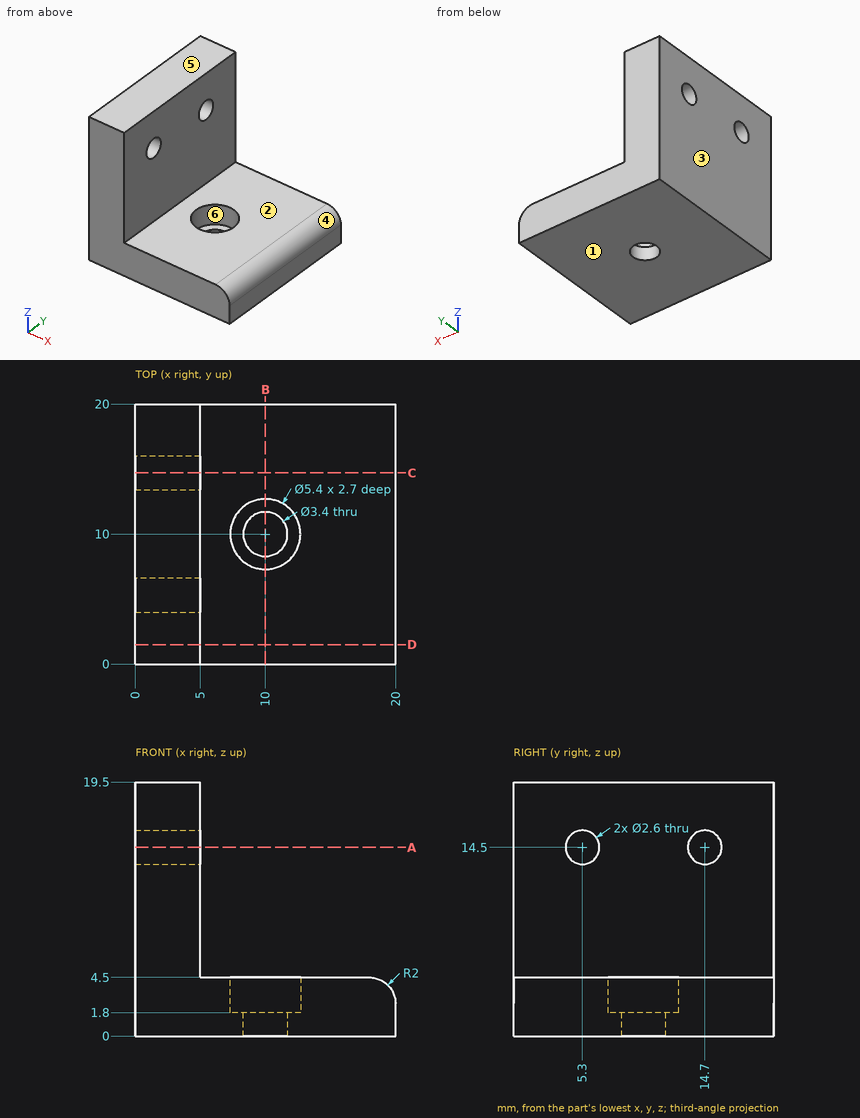
Answer from the drawing. Dimensions are ordinates in mm from the lowest x, y and z of the part. A direction names the side the tool comes from. Round coordinates to 2 decimals unless told otherwise and drop trailing zeros. Write each loop counter-clockwise with the first axis right and the second up, starting at its lowest first coordinate (ties: lowest second). Pieces come first, ordered by that corner, then holes. Notation, with made-up numbers: (-21, 67) - (0, 67) arc R29 cw to (0, 98) - close; hole circle Ø3 at (7, 48.25). An arc over 180 degrees is marked (long way). Use a Markdown table: item, result.
(1) Which of the six approach directions +Z, -Z, +X, -X, +Y, -Y give full straight-line access (tool end or side, diameter ignored) to the marked faces 1 and 2?
Reported:
| item | result |
|---|---|
| face 1 | -Z, +X, -X, +Y, -Y |
| face 2 | +Z, +X, +Y, -Y |
(2) The mould has two halves that part along X. Classify the marked faces 3, 4, 5 and 6: released by +X, released by -X, zero draft, split by the parting line, or undercut.
Reported:
| item | result |
|---|---|
| face 3 | released by -X |
| face 4 | released by +X |
| face 5 | zero draft |
| face 6 | undercut |
(3) The part is cut by section A-A (z = 14.5). Write down the section's boundary in (x, y).
Reported:
| item | result |
|---|---|
| outline | (0, 0) - (5, 0) - (5, 4) - (0, 4) - close; (0, 6.6) - (5, 6.6) - (5, 13.4) - (0, 13.4) - close; (0, 16) - (5, 16) - (5, 20) - (0, 20) - close |
(4) The part is cut by section D-D (y = 1.5). Write down the section's boundary in (x, z), then the cut area to 3 significant figures.
Reported:
| item | result |
|---|---|
| outline | (0, 0) - (20, 0) - (20, 2.5) arc R2 ccw to (18, 4.5) - (5, 4.5) - (5, 19.5) - (0, 19.5) - close |
| area | 164 mm2 |
(5) The part is cut by section B-B (x = 10). Write down the section's boundary in (y, z).
Reported:
| item | result |
|---|---|
| outline | (0, 0) - (8.3, 0) - (8.3, 1.8) - (7.3, 1.8) - (7.3, 4.5) - (0, 4.5) - close; (11.7, 0) - (20, 0) - (20, 4.5) - (12.7, 4.5) - (12.7, 1.8) - (11.7, 1.8) - close |
(6) The part is cut by section C-C (y = 14.7). Write down the section's boundary in (x, z), then the cut area to 3 significant figures.
Reported:
| item | result |
|---|---|
| outline | (0, 0) - (20, 0) - (20, 2.5) arc R2 ccw to (18, 4.5) - (5, 4.5) - (5, 13.2) - (0, 13.2) - close; (0, 15.8) - (5, 15.8) - (5, 19.5) - (0, 19.5) - close |
| area | 151 mm2 |
(7) Each of these flat-tipped pins is pushed along its axis until it touches: pin 1 Ø8 at (x, y) = (15.5, 13) entering from +Z; pin 2 Ø4 at (y, z) = (14.7, 14.5) entering from +X. Where does it stop, or does it pass through?
Reported:
| item | result |
|---|---|
| pin 1 | z = 4.5 |
| pin 2 | x = 5 |
(8) Straight lines are drawn through the part: line 1 along Z through (x, y) = (1.2, 5.3); line 2 along Z through (x, y) = (5.5, 6.75); line 3 along Z through (x, y) = (12.25, 11.25). For each, find the intervals that lie inside material, in ascending order. Write a range as [from, to].
Reported:
| item | result |
|---|---|
| line 1 | [0, 13.2], [15.8, 19.5] |
| line 2 | [0, 4.5] |
| line 3 | [0, 1.8] |
